from build123d import *

# Parameters (mm, degrees)
F0_R      = 38.1
F1_DEPTH  = 38.1
F1_FACE_R = 38.1
F2_DEPTH  = 38.1
F3_T      = -12.7


with BuildPart() as f1:
    # F0 (on Top) → F1 (new body)
    with BuildSketch(Plane.XY):
        Circle(F0_R)
    extrude(amount=-F1_DEPTH)

    # F1_face (on face) → F2 (join)
    with BuildSketch(Plane.XY):
        Circle(F1_FACE_R)
    extrude(amount=F2_DEPTH)

    # F3
    f3_openings = [f1.faces().sort_by_distance(p)[0] for p in [
        (0, 0, 38.1),
    ]]
    offset(amount=F3_T, openings=f3_openings)


solid = f1.part
CAD build for the part. Positions are in the model's coordinates, mm. Give positions to 0.01 mm unless a question says otherwise; leave off trailing zeros. Write each loop counter-clockwise with the first axis right and the second up, starting at its lowest first coordinate (ties: lowest second). Pieces come first, ordered by that corner, then holes. Notation, with made-up numbers: (27.5, 89.25) -> (57.5, 89.25) arc R16 cw to (57.5, 117.25) -> close; hole circle Ø5 at (87.5, 21). An arc over 180 degrees is marked (long way). Return JSON: item names as keys, results as strings.
Item 1: Band-saw the part on D-D (x = 32). List the corners of the cut face in (y, z), then the cut area to 3 significant figures.
Answer below:
{"outline": "(-20.68, -38.1) -> (20.68, -38.1) -> (20.68, 38.1) -> (-20.68, 38.1) -> close", "area": "3,150 mm2"}
Item 2: Drop flat-ended pins along their axis: pin 1 (6 mm diameter, centred on y = 5, z = -4.5, fed in from -X); pin 2 (5 mm diameter, centred on x = 0, z = -1, fed in from -Y); pin 3 (12 mm diameter, centred on y = 17, z = -12, fed in from +X). Give the stop position or say it passes through.
Answer below:
{"pin 1": "stops at x = -38.05", "pin 2": "stops at y = -38.1", "pin 3": "stops at x = 36.48"}
Item 3: Two-plate mould, pull along Y, no slides. Class faces 1 (the flat face through (-1, 1, -38.1)), 2 (the flat face through (0, 0, -25.4)): +Y half, -Y half, draft (parallel to the pull), parting line (faces both ways), or undercut.
Answer below:
{"face 1": "draft", "face 2": "undercut"}
Item 4: Drill centre lines: probe 1 along Y at (x, z) = (0, 9); probe 2 along Z at (x, y) = (-11, -10); probe 3 along Y at (x, z) = (-3, -8.5). Where is each one in solid material? Low to high.
Answer below:
{"probe 1": "y = -38.1 to -25.4, 25.4 to 38.1", "probe 2": "z = -38.1 to -25.4", "probe 3": "y = -37.98 to -25.22, 25.22 to 37.98"}
Item 5: Band-saw the part on A-A (x = 0). List the corners of the cut face in (y, z).
Answer below:
{"outline": "(-38.1, -38.1) -> (38.1, -38.1) -> (38.1, 38.1) -> (25.4, 38.1) -> (25.4, -25.4) -> (-25.4, -25.4) -> (-25.4, 38.1) -> (-38.1, 38.1) -> close"}
Item 6: Band-saw the part on C-C (z = 6). List the corners of the cut face in (x, y), then the cut area to 3 significant figures.
Answer below:
{"outline": "circle Ø76.2 at (0, 0); hole circle Ø50.8 at (0, 0)", "area": "2,530 mm2"}
